from build123d import *

# Parameters (mm, degrees)
SKETCH1_W             = 50.8
SKETCH1_H             = 76.2
BOSS_EXTRUDE1_DEPTH   = 975
SKETCH2_W             = 46.8
SKETCH2_H             = 72.2
CUT_EXTRUDE1_DEPTH    = 977.074674397
FILLET2_R             = 2
CROQUIS1_R            = 2.5
CORTAR_EXTRUIR1_DEPTH = 10
CROQUIS2_R            = 2.5
CORTAR_EXTRUIR2_DEPTH = 10
CROQUIS4_R            = 2.5
CORTAR_EXTRUIR3_DEPTH = 10
MATRIZL1_COUNT        = 17
MATRIZL1_PITCH        = 50


with BuildPart() as part:
    # Sketch1 → Boss-Extrude1 (new body)
    with BuildSketch(Plane(origin=(0, 0, 0), x_dir=(0, 0, -1), z_dir=(1, 0, 0))):
        Rectangle(SKETCH1_W, SKETCH1_H)
    extrude(amount=-BOSS_EXTRUDE1_DEPTH)

    # Sketch2 → Cut-Extrude1 (cut, through all)
    with BuildSketch(Plane(origin=(0, 0, 0), x_dir=(0, 0, -1), z_dir=(1, 0, 0))):
        Rectangle(SKETCH2_W, SKETCH2_H)
    extrude(amount=-CUT_EXTRUDE1_DEPTH, mode=Mode.SUBTRACT)

    # Fillet2
    fillet2_edges = [part.edges().sort_by_distance(p)[0] for p in [
        (-487.5, -36.1, 23.4),
        (-487.5, 36.1, 23.4),
        (-487.5, 36.1, -23.4),
        (-487.5, -36.1, -23.4),
        (-487.5, 38.1, 25.4),
        (-487.5, 38.1, -25.4),
        (-487.5, -38.1, -25.4),
        (-487.5, -38.1, 25.4),
    ]]
    fillet(fillet2_edges, radius=FILLET2_R)

    # Croquis1 → Cortar-Extruir1 (cut)
    with BuildSketch(Plane(origin=(0, 0, -25.4), x_dir=(-1, 0, 0), z_dir=(0, 0, -1))):
        with Locations(Location((25.4, 0, 0), (0, 0, 90))):
            Circle(CROQUIS1_R)
        with Locations(Location((10, 23.1, 0), (0, 0, 90))):
            Circle(CROQUIS1_R)
        with Locations(Location((10, -23.1, 0), (0, 0, 90))):
            Circle(CROQUIS1_R)
        with Locations(Location((40.8, -23.1, 0), (0, 0, 90))):
            Circle(CROQUIS1_R)
        with Locations(Location((40.8, 23.1, 0), (0, 0, 90))):
            Circle(CROQUIS1_R)
    extrude(amount=-CORTAR_EXTRUIR1_DEPTH, mode=Mode.SUBTRACT)

    # Croquis2 → Cortar-Extruir2 (cut)
    with BuildSketch(Plane(origin=(0, 0, -25.4), x_dir=(-1, 0, 0), z_dir=(0, 0, -1))):
        with Locations(Location((949.6, 0, 0), (0, 0, 90))):
            Circle(CROQUIS2_R)
        with Locations(Location((934.2, 23.1, 0), (0, 0, 90))):
            Circle(CROQUIS2_R)
        with Locations(Location((965, 23.1, 0), (0, 0, 90))):
            Circle(CROQUIS2_R)
        with Locations(Location((965, -23.1, 0), (0, 0, 90))):
            Circle(CROQUIS2_R)
        with Locations(Location((934.2, -23.1, 0), (0, 0, 90))):
            Circle(CROQUIS2_R)
    extrude(amount=-CORTAR_EXTRUIR2_DEPTH, mode=Mode.SUBTRACT)

    # Croquis4 → Cortar-Extruir3 (cut)
    with BuildSketch(Plane(origin=(0, 0, -25.4), x_dir=(-1, 0, 0), z_dir=(0, 0, -1))):
        with Locations(Location((87.5, 0, 0), (0, 0, 90))):
            Circle(CROQUIS4_R)
    cortar_extruir3 = extrude(amount=-CORTAR_EXTRUIR3_DEPTH, mode=Mode.SUBTRACT)

    # MatrizL1: Cortar-Extruir3 ×17
    with Locations(*[(-i * MATRIZL1_PITCH, 0, 0) for i in range(1, MATRIZL1_COUNT)]):
        add(cortar_extruir3, mode=Mode.SUBTRACT)


solid = part.part
Could you check a few things on this model? Use its own coordinates, in mm. A direction names the side the tool comes from. Give positions to 0.01 mm unless a question says otherwise; leave off trailing zeros. Loops run counter-clockwise (first coordinate to the right, second up) from the corner with the lowest first, then second, coordinate; pieces in that order, holes last. Notation, with made-up numbers: M 16.5,37 L 52.5,37 A26 cw 52.5,70 Z; hole C 12.5,87.25 d6. An arc over 180 degrees is marked long. Answer as a JSON object with one key per item and string values.
Q1. Suppose I cut it at B-B, the plane z = 2. List the corners of the cut face in (x, y) for me, plus the area to 3 significant figures.
Values found:
{"outline": "M -975,-38.1 L 0,-38.1 L 0,-36.1 L -975,-36.1 Z; M -975,36.1 L 0,36.1 L 0,38.1 L -975,38.1 Z", "area": "3,900 mm²"}
Q2. For P1, Ø4, axis at x = -587.5, y = 0, coming from the -Z side; P2, Ø8, axis at x = -965, y = 23.1, coming from the -Z side, each with a flat end and sliding along its axis, tell me the tip position at first contact or that it passes through.
Values found:
{"P1": "stops at z = 23.4", "P2": "stops at z = -25.4"}
Q3. If I drill on probe 1 along Z at (x, y) = (-498, -6); probe 2 along Y at (x, z) = (-887, -24); probe 3 along Y at (x, z) = (-153, 14.5), over which ranges is the centre line in solid material (lowest first)? Write a range as [from, to].
Values found:
{"probe 1": "z = [-25.4, -23.4], [23.4, 25.4]", "probe 2": "y = [-38.01, -2.45], [2.45, 38.01]", "probe 3": "y = [-38.1, -36.1], [36.1, 38.1]"}
Q4. For faces 1 (the flat face through (-481, 0, 23.4)), 2 (the flat face through (-481, -1, 25.4)), which set-ups out of +Z, -Z, +X, -X, +Y, -Y let a thin tool reach every point of the face, with its end or its side?
Values found:
{"face 1": "+X, -X", "face 2": "+Z, +X, -X, +Y, -Y"}
Q5. Suppose I cut it at A-A, the plane x = -173. List the corners of the cut face in (y, z) for me, plus the area to 3 significant figures.
Values found:
{"outline": "M -38.1,-23.4 A2 ccw -36.1,-25.4 L 36.1,-25.4 A2 ccw 38.1,-23.4 L 38.1,23.4 A2 ccw 36.1,25.4 L -36.1,25.4 A2 ccw -38.1,23.4 Z; hole M -36.1,-21.4 A2 ccw -34.1,-23.4 L 34.1,-23.4 A2 ccw 36.1,-21.4 L 36.1,21.4 A2 ccw 34.1,23.4 L -34.1,23.4 A2 ccw -36.1,21.4 Z", "area": "492 mm²"}
